Model file for the job. Use its own axes, mm. Face numbers are marked on the shaded views. A direction names the side the tool comes from. Round coordinates to 2 decimals unless told otherwise and drop trailing zeros. Order: outer loops, then holes, each group sorted by start corner. A loop starts at its lowest first (then second) coordinate and runs counter-clockwise, first axis right, second up. Notation, with made-up numbers: (66, 31) - (71, 31) arc R30 cw to (71, 65) - close; hole circle Ø3 at (10.5, 29.25). An arc over 180 degrees is marked (long way). Answer as CSV lines item,"result". Start each with the question number.
1. Pull direction X, two halves, no side cores. Call the marked faces 3, 4 and 5: released by +X, released by -X, zero draft, split by the parting line, or undercut.
2. Wall check: line 1 along Z through (x, y) = (-7.62, 15); line 2 along Z through (x, y) = (-13, 21); line 3 along Z through (x, y) = (22, 18.25). Give the ranges that are in metal, low to high. Write a range as [from, to].
3. Band-saw the part on B-B on x = -12.7. List the corners of the cut face in (y, z) (3 decimals), then the cut area to 3 significant figures.
4. 3-axis set-ups, long thin cutter, end or side, ignore diameter. For the marked faces 1 and 2: which of +Z, -Z, +X, -X, +Y, -Y reach the whole face in a straight line?
5. Pin check, flat tips, straight feed: pin 1 Ø1.4 at (x, z) = (-10.16, -27.94) entering from -Y; pin 2 Ø4 at (x, z) = (-31.75, -15.875) entering from +Y. Stop position of each tip, or through.
6. Band-saw the part on C-C on y = 2.25. State how many separate pieces and enclosed holes the cut face has, then the cut area to 3 significant figures.
7. Band-saw the part on A-A on z = 6. List the corners of the cut face in (x, y) (3 decimals), then the cut area to 3 significant figures.
```python
from build123d import *

# Parameters (mm, degrees)
SKETCH1_W                       = 76.2
SKETCH1_H                       = 76.2
BOSS_EXTRUDE1_DEPTH             = 22.225
SKETCH2_W                       = 44.45
SKETCH2_H                       = 38.1
CUT_EXTRUDE1_DEPTH              = 59.285252208
CUT_EXTRUDE2_DEPTH              = 59.285252208
F_3_32_0_09375_DIAMETER_HOLE1_D = 2.38125
CUT_EXTRUDE4_DEPTH              = 21.59
CUT_EXTRUDE5_REACH              = 79.316
CHAMFER1_SIZE                   = 0.762
CHAMFER2_SIZE                   = 0.508
F_1_4_0_25_DIAMETER_HOLE1_D     = 6.35
F_1_4_0_25_DIAMETER_HOLE1_DEPTH = 16.51
F_1_4_0_25_DIAMETER_HOLE1_TIP   = 1.907732465


with BuildPart() as part:
    # Sketch1 → Boss-Extrude1 (new body)
    with BuildSketch(Plane(origin=(0, 0, 0), x_dir=(1, 0, 0), z_dir=(0, 1, 0))):
        Rectangle(SKETCH1_W, SKETCH1_H)
    extrude(amount=BOSS_EXTRUDE1_DEPTH)

    # Sketch2 → Cut-Extrude1 (cut, through all)
    with BuildSketch(Plane(origin=(0, 22.225, 0), x_dir=(1, 0, 0), z_dir=(0, 1, 0))):
        Rectangle(SKETCH2_W, SKETCH2_H)
    extrude(amount=-CUT_EXTRUDE1_DEPTH, mode=Mode.SUBTRACT)

    # Sketch3 → Cut-Extrude2 (cut, through all)
    with BuildSketch(Plane(origin=(0, 22.225, 0), x_dir=(1, 0, 0), z_dir=(0, 1, 0))):
        with BuildLine():
            Line((-19.05, 19.05), (-19.05, -19.05))
            ThreePointArc((-19.05, -19.05), (-22.225, -22.225), (-25.4, -19.05))
            Line((-25.4, -19.05), (-25.4, 19.05))
            ThreePointArc((-25.4, 19.05), (-22.225, 22.225), (-19.05, 19.05))
        make_face()
        with BuildLine():
            Line((25.4, 19.05), (25.4, -19.05))
            ThreePointArc((25.4, -19.05), (22.225, -22.225), (19.05, -19.05))
            Line((19.05, -19.05), (19.05, 19.05))
            ThreePointArc((19.05, 19.05), (22.225, 22.225), (25.4, 19.05))
        make_face()
    extrude(amount=-CUT_EXTRUDE2_DEPTH, mode=Mode.SUBTRACT)

    # 3/32 (0.09375) Diameter Hole1 (through all)
    with Locations(Plane(origin=(0, 22.225, 0), x_dir=(1, 0, 0), z_dir=(0, 1, 0))):
        with Locations((-15.24, 27.94), (15.24, 27.94), (-17.78, 33.02), (17.78, 33.02), (-12.7, 33.02), (-7.62, 33.02), (-2.54, 33.02), (2.54, 33.02), (7.62, 33.02), (12.7, 33.02), (-10.16, 27.94), (-5.08, 27.94), (0, 27.94), (5.08, 27.94), (10.16, 27.94)):
            f_3_32_0_09375_diameter_hole1 = Hole(F_3_32_0_09375_DIAMETER_HOLE1_D / 2)

    # Mirror1: 3/32 (0.09375) Diameter Hole1 across plane
    add(f_3_32_0_09375_diameter_hole1.mirror(Plane.XY), mode=Mode.SUBTRACT)

    # Sketch8 → Cut-Extrude4 (cut, symmetric)
    with BuildSketch(Plane(origin=(0, 0, 0), x_dir=(0, 0, -1), z_dir=(1, 0, 0))):
        Polygon((19.304, 22.225), (20.32, 21.209), (21.336, 22.225), align=None)
    cut_extrude4 = extrude(amount=CUT_EXTRUDE4_DEPTH, both=True, mode=Mode.SUBTRACT)

    # Mirror2: Cut-Extrude4 across plane
    add(cut_extrude4.mirror(Plane.XY), mode=Mode.SUBTRACT)

    # Sketch9 → Cut-Extrude5 (cut, up to next)
    with BuildSketch(Plane(origin=(-25.4, 0, 0), x_dir=(0, 0, -1), z_dir=(1, 0, 0)), mode=Mode.PRIVATE) as cut_extrude5_sk1:
        with BuildLine():
            Line((3.175, 15.875), (3.175, 9.525))
            ThreePointArc((3.175, 9.525), (0, 6.35), (-3.175, 9.525))
            Line((-3.175, 9.525), (-3.175, 15.875))
            ThreePointArc((-3.175, 15.875), (0, 19.05), (3.175, 15.875))
        make_face()
    cut_extrude5_tool1 = extrude(cut_extrude5_sk1.sketch, amount=-CUT_EXTRUDE5_REACH, mode=Mode.PRIVATE) & part.part
    add(cut_extrude5_tool1.solids().sort_by_distance((-25.4, 12.7, 0))[0], mode=Mode.SUBTRACT)

    # Chamfer1
    chamfer1_edges = [part.edges().sort_by_distance(p)[0] for p in [
        (-38.1, 22.225, 0),
        (0, 22.225, 38.1),
        (38.1, 22.225, 0),
        (0, 0, 38.1),
        (-38.1, 0, 0),
        (0, 0, -38.1),
        (38.1, 0, 0),
        (0, 22.225, -38.1),
    ]]
    chamfer(chamfer1_edges, length=CHAMFER1_SIZE)

    # Chamfer2
    chamfer2_edges = [part.edges().sort_by_distance(p)[0] for p in [
        (-25.4, 19.05, 0),
        (-25.4, 12.7, 3.175),
        (-25.4, 6.35, 0),
        (-25.4, 12.7, -3.175),
        (-38.1, 12.7, 3.175),
        (-38.1, 19.05, 0),
        (-38.1, 12.7, -3.175),
        (-38.1, 6.35, 0),
    ]]
    chamfer(chamfer2_edges, length=CHAMFER2_SIZE)

    # 1/4 (0.25) Diameter Hole1
    with Locations(Plane(origin=(0, 22.225, 0), x_dir=(1, 0, 0), z_dir=(0, 1, 0))):
        with Locations((-31.75, 15.875), (-31.75, -15.875)):
            Hole(F_1_4_0_25_DIAMETER_HOLE1_D / 2, depth=F_1_4_0_25_DIAMETER_HOLE1_DEPTH)
            with Locations((0, 0, -(F_1_4_0_25_DIAMETER_HOLE1_DEPTH + F_1_4_0_25_DIAMETER_HOLE1_TIP / 2))):  # 118° drill point
                Cone(0, F_1_4_0_25_DIAMETER_HOLE1_D / 2, F_1_4_0_25_DIAMETER_HOLE1_TIP, mode=Mode.SUBTRACT)


solid = part.part
```
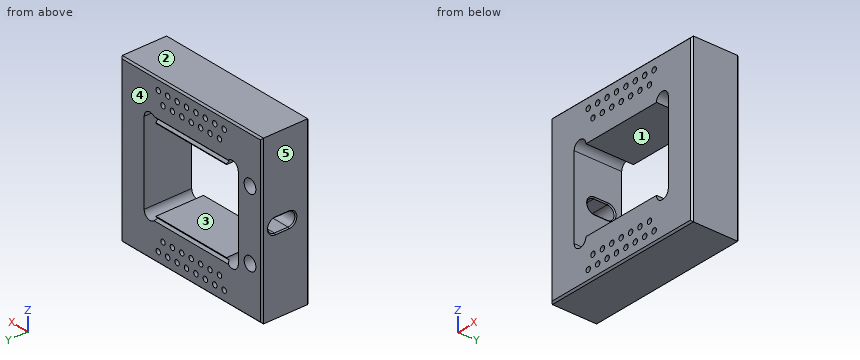
Reply:
1,face 3,"undercut"
1,face 4,"zero draft"
1,face 5,"released by -X"
2,line 1,"z = [-38.1, -34.21], [-31.83, -19.05], [19.05, 31.83], [34.21, 38.1]"
2,line 2,"z = [-38.1, -34.17], [-31.87, -19.05], [19.05, 31.87], [34.17, 38.1]"
2,line 3,"z = [-38.1, -22.22], [22.22, 38.1]"
3,outline,"(0, -37.338) - (0.762, -38.1) - (21.463, -38.1) - (22.225, -37.338) - (22.225, -34.211) - (0, -34.211) - close; (0, -31.829) - (22.225, -31.829) - (22.225, -21.336) - (21.209, -20.32) - (22.225, -19.304) - (22.225, -19.05) - (0, -19.05) - close; (0, 19.05) - (22.225, 19.05) - (22.225, 19.304) - (21.209, 20.32) - (22.225, 21.336) - (22.225, 31.829) - (0, 31.829) - close; (0, 34.211) - (22.225, 34.211) - (22.225, 37.338) - (21.463, 38.1) - (0.762, 38.1) - (0, 37.338) - close"
3,area,"738 mm2"
4,face 1,"+Y, -Y"
4,face 2,"+Z, +X, -X, +Y, -Y"
5,pin 1,"passes through"
5,pin 2,"stops at y = 5.01"
6,separate pieces,"1"
6,enclosed holes,"31"
6,area,"3,670 mm2"
7,outline,"(-38.1, 0.762) - (-37.338, 0) - (-25.4, 0) - (-25.4, 22.225) - (-37.338, 22.225) - (-38.1, 21.463) - close; (25.4, 0) - (37.338, 0) - (38.1, 0.762) - (38.1, 21.463) - (37.338, 22.225) - (25.4, 22.225) - close"
7,area,"563 mm2"
